from build123d import *

# Parameters (mm, degrees)
F0_W     = 101.6
F0_H     = 38.1
F1_DEPTH = 3.175
F3_DEPTH = 254
F2_R     = 3.81
F2_R_2   = 3.175
F4_DEPTH = 101.6


with BuildPart() as f1:
    # F0 (on Top) → F1 (new body)
    with BuildSketch(Plane.XY):
        with Locations((-50.8, -19.05)):
            Rectangle(F0_W, F0_H)
    extrude(amount=F1_DEPTH)

    # F2 (on face) → F3 (cut)
    with BuildSketch(Plane(origin=(-101.6, 0, 0), x_dir=(0, -1, 0), z_dir=(-1, 0, 0))):
        with BuildLine():
            ThreePointArc((3.7567106623, 3.175), (3.7966542918, 3.4913839483), (3.81, 3.81))
            ThreePointArc((3.81, 3.81), (-2.6940768363, 6.5040768363), (0, 0))
            Line((0, 0), (0, 0.635))
            ThreePointArc((0, 0.635), (-2.2450640303, 6.0550640303), (3.175, 3.81))
            ThreePointArc((3.175, 3.81), (3.1589222858, 3.4908840456), (3.1108519733, 3.175))
            Line((3.1108519733, 3.175), (3.7567106623, 3.175))
        make_face()
        with BuildLine():
            Line((0, 0.635), (0, 0))
            ThreePointArc((0, 0), (2.4593444248, 0.9000644337), (3.7567106623, 3.175))
            Line((3.7567106623, 3.175), (3.1108519733, 3.175))
            ThreePointArc((3.1108519733, 3.175), (2.0080463142, 1.3506555752), (0, 0.635))
        make_face()
        with BuildLine():
            Line((0, 3.175), (0, 0.635))
            ThreePointArc((0, 0.635), (2.0080463142, 1.3506555752), (3.1108519733, 3.175))
            Line((3.1108519733, 3.175), (0, 3.175))
        make_face()
    extrude(amount=-F3_DEPTH, mode=Mode.SUBTRACT)

    # F2 (on face) → F4 (join, through all)
    with BuildSketch(Plane(origin=(-101.6, 0, 0), x_dir=(0, -1, 0), z_dir=(-1, 0, 0))):
        with Locations((0, 3.81)):
            Circle(F2_R)
        with Locations((0, 3.81)):
            Circle(F2_R_2, mode=Mode.SUBTRACT)
    extrude(amount=-F4_DEPTH)


solid = f1.part
Could you check a few things on this model? Use its own coordinates, in mm. Round coordinates to 2 decimals unless told otherwise and drop trailing zeros. Write each loop counter-clockwise with the first axis right and the second up, starting at its lowest first coordinate (ties: lowest second). Pieces come first, ordered by that corner, then holes. Notation, with made-up numbers: (68, -16) -> (113, -16) arc R17 ccw to (113, 12) -> close; hole circle Ø3 at (-8.75, -9.75). An arc over 180 degrees is marked (long way). Use a Markdown table: item, result.
1. If we section it at B-B (z = 5): List the corners of the cut face in (x, y) for me, then the cut area to 3 significant figures.
Answer key:
| item | result |
|---|---|
| outline | (-101.6, -3.62) -> (0, -3.62) -> (0, -2.94) -> (-101.6, -2.94) -> close; (-101.6, 2.94) -> (0, 2.94) -> (0, 3.62) -> (-101.6, 3.62) -> close |
| area | 137 mm^2 |
2. Please list where these lines run through material, in increasing order: probe 1 along Y at (x, z) = (-62, 3.75); probe 2 along Z at (x, y) = (-65, 0) (3 decimals); probe 3 along Z at (x, y) = (-62, -7) (3 decimals).
Answer key:
| item | result |
|---|---|
| probe 1 | y = -3.81 to -3.17, 3.17 to 3.81 |
| probe 2 | z = 0 to 0.635, 6.985 to 7.62 |
| probe 3 | z = 0 to 3.175 |
3. For pin 1 Ø1 at (x, z) = (-43.5, 4.5) entering from +Y; pin 2 Ø10.5 at (x, y) = (-74.5, -19) entering from +Z (3 decimals), each with a flat end and sliding along its axis, tell me the tip position at first contact or that it passes through.
Answer key:
| item | result |
|---|---|
| pin 1 | stops at y = 3.81 |
| pin 2 | stops at z = 3.175 |
4. If we section it at A-A (x = -84): List the corners of the cut face in (y, z) for me (3 decimals).
Answer key:
| item | result |
|---|---|
| outline | (-38.1, 0) -> (0, 0) arc R3.81 ccw (long way) to (-3.757, 3.175) -> (-38.1, 3.175) -> close; hole circle Ø6.35 at (0, 3.81) |
5. We'd pull the mould along Y, two halves only. Please class faces 1 (the face through (-51.51, 0.69, 0.71)), 2 (the face through (0, -17, 2)), 3 (the face through (-52, -38.1, 2)): +Y half, -Y half, draft (parallel to the pull), parting line (faces both ways), or undercut.
Answer key:
| item | result |
|---|---|
| face 1 | undercut |
| face 2 | draft |
| face 3 | -Y half |
6. If we section it at C-C (y = -13): List the corners of the cut face in (x, z) for me (3 decimals).
Answer key:
| item | result |
|---|---|
| outline | (-101.6, 0) -> (0, 0) -> (0, 3.175) -> (-101.6, 3.175) -> close |
